Can you work these out from the drawing? Everything is in mm from the part's minimum corner. Coordinates: 2 decimals unless noted, no trailing zeros. Order: outer loops, then holes, each group sorted by start corner. A loop starts at its lowest first (then second) coordinate and runs counter-clockwise, first axis right, second up. Notation, with made-up numbers: M -39,74 L -3,74 A8 cw -3,79 Z; hole C 54,18.5 d8. An arc over 180 degrees is marked long. Answer as CSV lines item,"result". Start each with the question number.
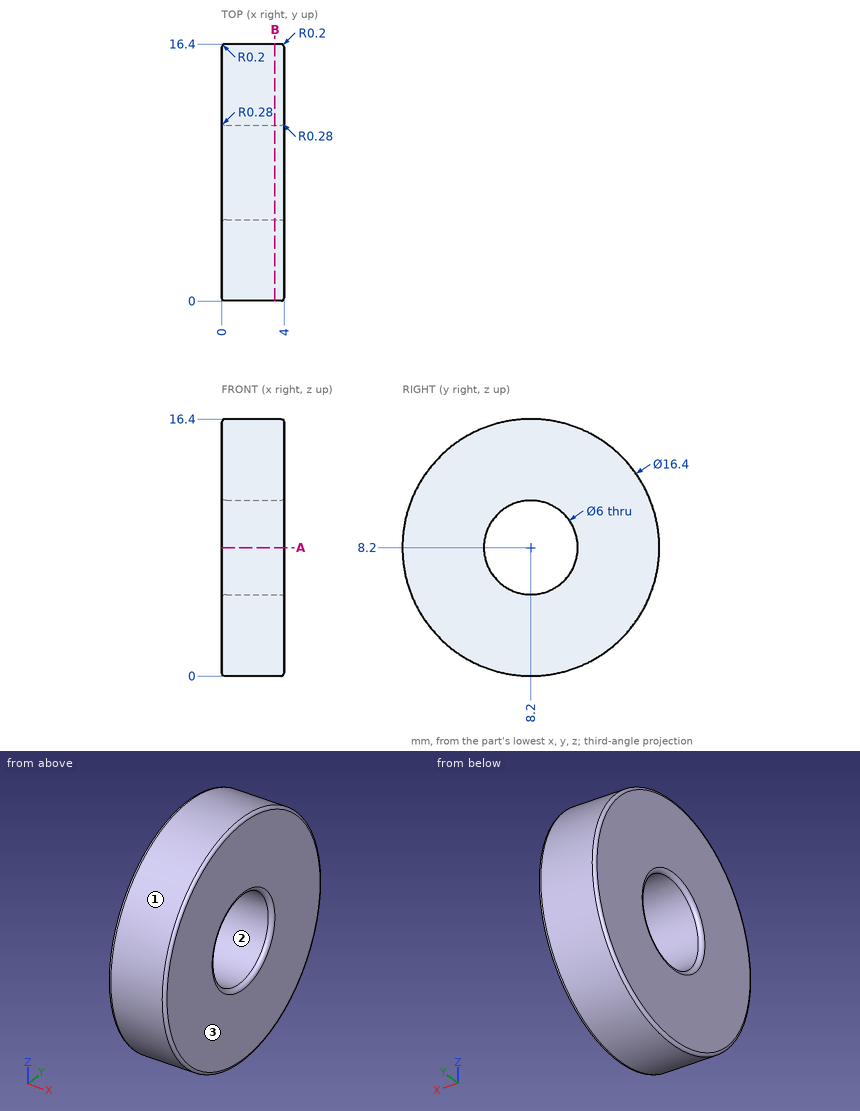
1) If we mould it in two halves opening along Z, with no side actions, what happens to the marked faces 1, 2 and 3? For each: released by +Z, released by -Z, zero draft, split by the parting line, or undercut.
2) Suppose I cut it at B-B on x = 3.4. Please give me the cut outline in (y, z), plus the area to 3 significant figures.
3) Will these pins go through, and if not, where does the flat tip stop? pin 1 Ø1.5 at (x, z) = (3, 2) entering from +Y; pin 2 Ø3.5 at (y, z) = (8.2, 8.2) entering from -X.
4) Suppose I cut it at A-A on z = 8.2. Please give me the cut outline in (x, y).
5) I need wall thicknesses on line 1 (Z direction, x = 2.55, y = 8.2); line 2 (Y direction, x = 0.75, z = 5.5); line 3 (Y direction, x = 2.9, z = 7.5). Which ranges of each line are inside material? Lowest first, please. Write a range as [from, to].
Output:
1,face 1,"split by the parting line"
1,face 2,"undercut"
1,face 3,"zero draft"
2,outline,"C 8.2,8.2 d16.4; hole C 8.2,8.2 d6"
2,area,"183 mm²"
3,pin 1,"y = 14.33"
3,pin 2,"through"
4,outline,"M 0,0.2 A0.2 ccw 0.2,0 L 3.8,0 A0.2 ccw 4,0.2 L 4,4.92 A0.28 ccw 3.72,5.2 L 0.28,5.2 A0.28 ccw 0,4.92 Z; M 0,11.48 A0.28 ccw 0.28,11.2 L 3.72,11.2 A0.28 ccw 4,11.48 L 4,16.2 A0.2 ccw 3.8,16.4 L 0.2,16.4 A0.2 ccw 0,16.2 Z"
5,line 1,"[0, 5.2], [11.2, 16.4]"
5,line 2,"[0.46, 6.89], [9.51, 15.94]"
5,line 3,"[0.03, 5.28], [11.12, 16.37]"
